from build123d import *

# Parameters (mm, degrees)
CROQUIS1_W                = 21
CROQUIS1_H                = 40
CROQUIS1_R                = 1.65
SALIENTE_EXTRUIR1_DEPTH   = 5
SALIENTE_EXTRUIR1_2_DEPTH = 5
CROQUIS1_3_W              = 48
CROQUIS1_3_H              = 40
CROQUIS1_3_R              = 3.175
SALIENTE_EXTRUIR2_DEPTH   = 18
CORTAR_EXTRUIR1_DEPTH     = 52
CHAFL_N1_SIZE2            = 13
CHAFL_N1_SIZE             = 5
CHAFL_N2_SIZE2            = 13
CHAFL_N2_SIZE             = 5
REDONDEO1_R               = 3
REDONDEO2_R               = 3


with BuildPart() as part:
    # Croquis1 → Saliente-Extruir1 (new body)
    with BuildSketch(Plane(origin=(0, 0, 0), x_dir=(1, 0, 0), z_dir=(0, 1, 0))):
        with Locations((-34.5, 0)):
            Rectangle(CROQUIS1_W, CROQUIS1_H)
        with Locations(Location((-41, -16, 0), (0, 0, 270))):
            Circle(CROQUIS1_R, mode=Mode.SUBTRACT)
        with Locations(Location((-41, 16, 0), (0, 0, 270))):
            Circle(CROQUIS1_R, mode=Mode.SUBTRACT)
    extrude(amount=SALIENTE_EXTRUIR1_DEPTH)



with BuildPart() as body_2:
    # Croquis1 → Saliente-Extruir1 2 (new body)
    with BuildSketch(Plane(origin=(0, 0, 0), x_dir=(1, 0, 0), z_dir=(0, 1, 0))):
        with Locations((34.5, 0)):
            Rectangle(CROQUIS1_W, CROQUIS1_H)
        with Locations(Location((41, -16, 0), (0, 0, 270))):
            Circle(CROQUIS1_R, mode=Mode.SUBTRACT)
        with Locations(Location((41, 16, 0), (0, 0, 270))):
            Circle(CROQUIS1_R, mode=Mode.SUBTRACT)
    extrude(amount=SALIENTE_EXTRUIR1_2_DEPTH)


with BuildPart() as part_1:
    add(part.part)

    add(body_2.part)  # Saliente-Extruir2 merges body 2
    # Croquis1<3> → Saliente-Extruir2 (add)
    with BuildSketch(Plane(origin=(0, 0, 0), x_dir=(1, 0, 0), z_dir=(0, 1, 0))):
        Rectangle(CROQUIS1_3_W, CROQUIS1_3_H)
        with Locations(Location((0, 0, 0), (0, 0, 270))):
            Circle(CROQUIS1_3_R, mode=Mode.SUBTRACT)
    extrude(amount=SALIENTE_EXTRUIR2_DEPTH)

    # Croquis2 → Cortar-Extruir1 (cut)
    with BuildSketch(Plane.XY.offset(20)):
        with BuildLine():
            Line((-17.262904506, 9.533811896), (17.262904506, 9.533811896))
            add(Edge.make_bspline(
                [(22.266442187, 18), (22.701537977, 9.819720853), (17.262904506, 9.533811896)],
                knots=[0, 0, 0, 1, 1, 1], degree=2))
            Line((22.266442187, 18), (-22.266442187, 18))
            add(Edge.make_bspline(
                [(-22.266442187, 18), (-22.701537977, 9.819720853), (-17.262904506, 9.533811896)],
                knots=[0, 0, 0, 1, 1, 1], degree=2))
        make_face()
    extrude(amount=-CORTAR_EXTRUIR1_DEPTH, mode=Mode.SUBTRACT)

    # Chaflán1
    chafl_n1_edges = [part_1.edges().sort_by_distance(p)[0] for p in [
        (-24, 5, 0),
    ]]
    chafl_n1_side = [part_1.faces().sort_by_distance(p)[0] for p in [
        (-24.1, 5, 0),
    ]]
    chamfer(chafl_n1_edges, length=CHAFL_N1_SIZE - 0.0001, length2=CHAFL_N1_SIZE2 - 0.0001, reference=chafl_n1_side[0])  # a hair under: the kernel refuses the full size

    # Chaflán2
    chafl_n2_edges = [part_1.edges().sort_by_distance(p)[0] for p in [
        (24, 5, 0),
    ]]
    chafl_n2_side = [part_1.faces().sort_by_distance(p)[0] for p in [
        (24.1, 5, 0),
    ]]
    chamfer(chafl_n2_edges, length=CHAFL_N2_SIZE - 0.0001, length2=CHAFL_N2_SIZE2 - 0.0001, reference=chafl_n2_side[0])  # a hair under: the kernel refuses the full size

    # Redondeo1
    redondeo1_edges = [part_1.edges().sort_by_distance(p)[0] for p in [
        (-28.9999, 5, 0),
        (28.9999, 5, 0),
    ]]
    fillet(redondeo1_edges, radius=REDONDEO1_R)

    # Redondeo2
    redondeo2_edges = [part_1.edges().sort_by_distance(p)[0] for p in [
        (-45, 2.5, 20),
        (-45, 2.5, -20),
        (45, 2.5, -20),
        (45, 2.5, 20),
    ]]
    fillet(redondeo2_edges, radius=REDONDEO2_R)


solid = part_1.part
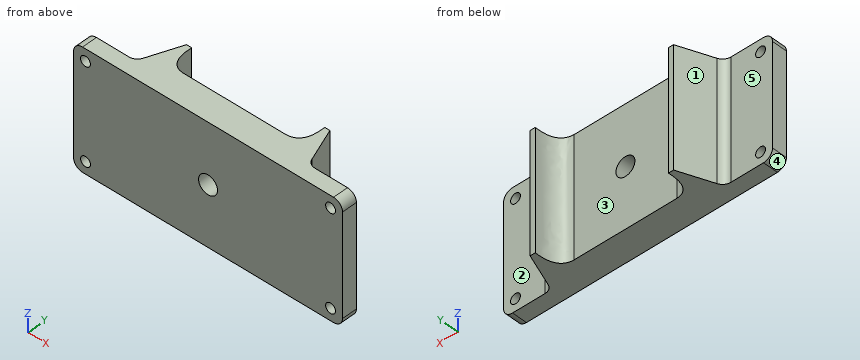
Can you work these out from the model? Positions are in its coordinate system, mm. Face numbers are marked on the shaded views. A direction names the side the tool comes from. Give positions to 0.01 mm unless a question says otherwise; leave off trailing zeros. Order: outer loops, then holes, each group sorted by start corner. A loop starts at its lowest first (then second) coordinate and runs counter-clockwise, first axis right, second up. Notation, with made-up numbers: M -16.75,35 L -6.75,35 A33 ccw -6.75,71 Z; hole C 1,15.5 d7. An arc over 180 degrees is marked long. Use a Markdown table: item, result. Add a question column.
Item 1: For the marked faces 4 and 5, which set-ups out of +Z, -Z, +X, -X, +Y, -Y let a thin tool reach every point of the face, with its end or its side?
Item 2: Suppose I cut it at D-D (z = -16). Count the separate pieces of the cut face and the enclosed holes in it, then the cut area to 3 significant figures.
Item 3: Suppose I cut it at A-A (x = -41). List the corners of the cut face in (y, z) for me, then the cut area to 3 significant figures.
Item 4: Suppose I cut it at B-B (x = 0). List the corners of the cut face in (y, z) for me (3 decimals), then the cut area to 3 significant figures.
Item 5: Suppose I cut it at C-C (y = 8.5). List the corners of the cut face in (x, z) for me (3 decimals), then the cut area to 3 significant figures.
Item 6: Will these pins go through, and if not, where does the flat tip stop? pin 1 (1.5 mm diameter, centred on y = 6, z = -8.5, fed in from -X); pin 2 (4 mm diameter, centred on y = 15, z = -15.5, fed in from -X); pin 3 (3 mm diameter, centred on y = 8, z = 6, fed in from -X).
Item 7: We'd pull the mould along X, two halves only. Please class the marked faces 1, 2 and 3: +X half, -X half, draft (parallel to the pull), parting line (faces both ways), or undercut.
Item 8: If I drill on L1, parallel to X at y = 1.2, z = -16; L2, parallel to Y at x = 37, z = -8.5; L3, parallel to Z at x = 0, y = 7 (3 decimals), over which ranges is the centre line in solid material (lowest first)? Write a range as [from, to].
Answer sheet:
| question | item | result |
|---|---|---|
| 1 | face 4 | -Z, -X, +Y, -Y |
| 1 | face 5 | +Z, -Z, -X, +Y |
| 2 | separate pieces | 3 |
| 2 | enclosed holes | 0 |
| 2 | area | 743 mm² |
| 3 | outline | M 0,-20 L 5,-20 L 5,-17.65 L 0,-17.65 Z; M 0,-14.35 L 5,-14.35 L 5,14.35 L 0,14.35 Z; M 0,17.65 L 5,17.65 L 5,20 L 0,20 Z |
| 3 | area | 167 mm² |
| 4 | outline | M 0,-20 L 9.534,-20 L 9.534,-3.175 L 0,-3.175 Z; M 0,3.175 L 9.534,3.175 L 9.534,20 L 0,20 Z |
| 4 | area | 321 mm² |
| 5 | outline | M -27.654,-20 L 27.654,-20 L 27.654,20 L -27.654,20 Z; hole C 0,0 d6.35 |
| 5 | area | 2,180 mm² |
| 6 | pin 1 | stops at x = -29.86 |
| 6 | pin 2 | stops at x = -25.92 |
| 6 | pin 3 | stops at x = -28.46 |
| 7 | face 1 | -X half |
| 7 | face 2 | draft |
| 7 | face 3 | undercut |
| 8 | L1 | x = [-45, -42.65], [-39.35, 39.35], [42.65, 45] |
| 8 | L2 | y = [0, 5] |
| 8 | L3 | z = [-20, -3.175], [3.175, 20] |
